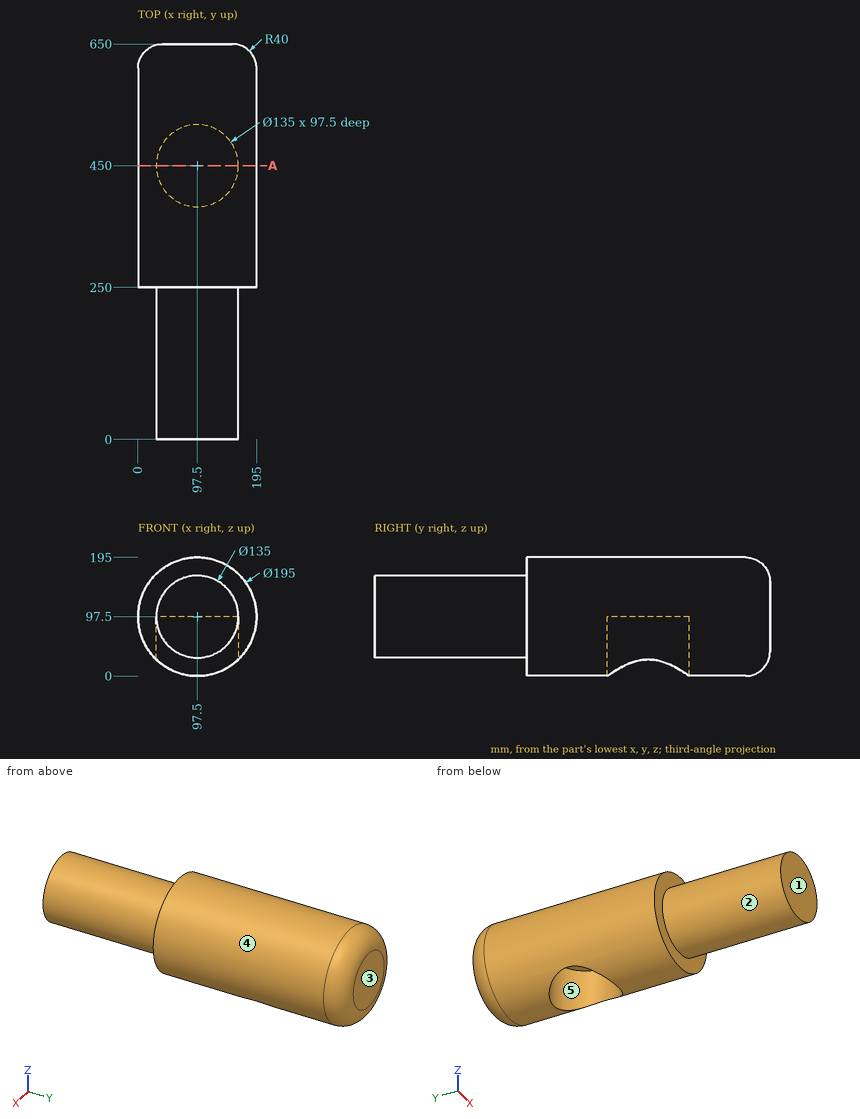
Here's the drawing with two shaded views (mm, measured from the low corner). I have some questions. A direction names the side the tool comes from. Give positions to 0.01 mm unless a question says otherwise; leave off trailing zeros. Loops run counter-clockwise (first coordinate to the right, second up) from the corner with the lowest first, then second, coordinate; pieces in that order, holes last. Notation, with made-up numbers: (15, -1.5) -> (38, -1.5) arc R4 ccw to (38, 5.5) -> close; hole circle Ø10 at (30, 80.5). An arc over 180 degrees is marked (long way). One line per item, written item: value.
Q1. I'm going to push flat-ended pins straight in: pin 1 Ø10 at (x, y) = (94.5, 576.5) entering from -Z; pin 2 Ø5 at (x, y) = (93, 424) entering from +Z; pin 3 Ø4 at (y, z) = (547, 143.5) entering from -X. Where does each tip first touch, or does it pass through?
Answers follow:
pin 1: z = 0
pin 2: z = 194.98
pin 3: x = 10.49
Q2. Suppose I cut it at A-A on y = 450. Please give me the cut outline in (x, z).
Answers follow:
outline: (30, 27.14) -> (30, 97.5) -> (165, 97.5) -> (165, 27.14) arc R97.5 ccw (long way) to start
Q3. If I drill on line 1 along Y through (x, z) = (97, 51); line 2 along Y through (x, z) = (128.5, 75); line 3 along X through (y, z) = (610.5, 100), over which ranges is the centre line in solid material (lowest first)?
Answers follow:
line 1: 0 to 382.5, 517.5 to 650
line 2: 0 to 390.04, 509.96 to 650
line 3: 0.04 to 194.96
Q4. We'd pull the mould along X, two halves only. Please class the marked faces 3, 4 and 5: pulls with the +X half, pulls with the -X half, needs draft (parallel to the pull), parting line crosses it, or undercut.
Answers follow:
face 3: needs draft
face 4: parting line crosses it
face 5: undercut
Q5. On a 3-axis mill with a long thin cutter (end or side, diameter ignored), from which of +Z, -Z, +X, -X, +Y, -Y can I reach the whole of each face in a straight line? I mean the marked faces 1 and 2. Say none if no direction works.
Answers follow:
face 1: +Z, -Z, +X, -X, -Y
face 2: -Y
